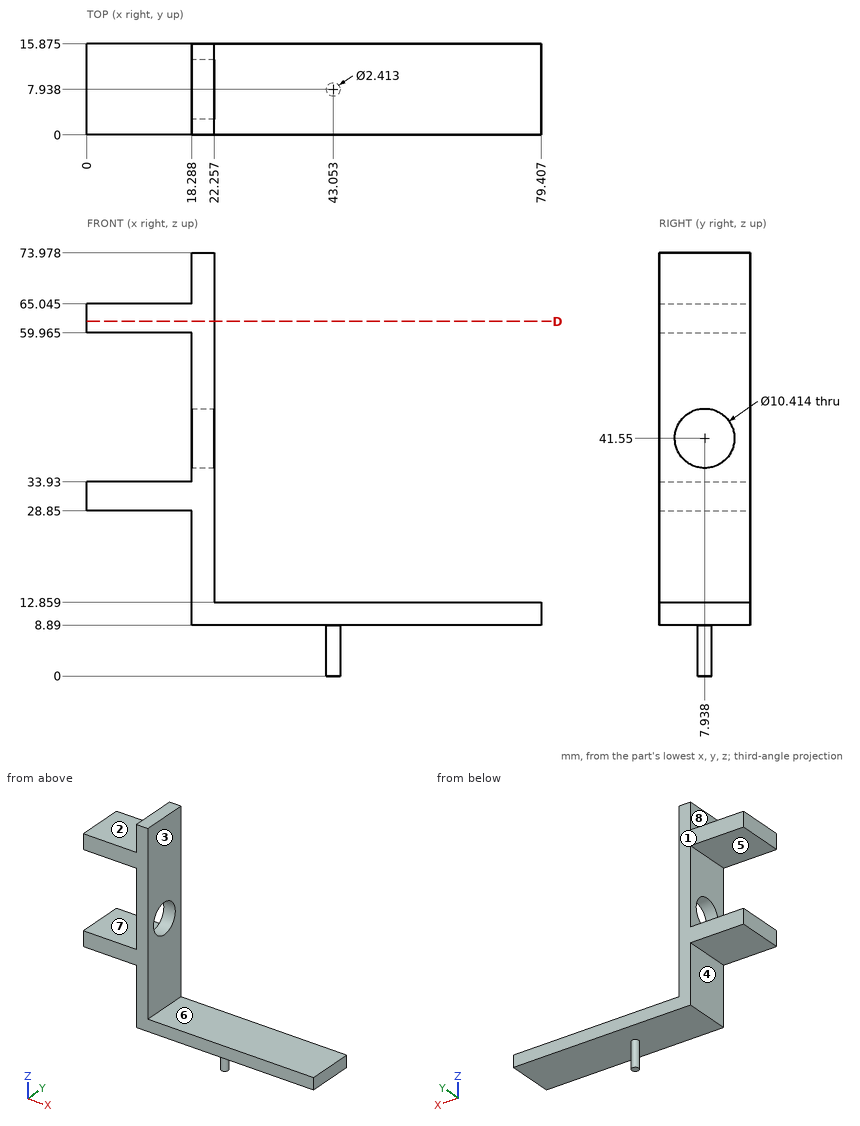
Design review of the part shown in the three views and the two pictorial views. Dimensions are in mm from the part's minimum x, y and z. A direction names the side the tool comes from. Round coordinates to 2 decimals unless told otherwise and drop trailing zeros. Loops run counter-clockwise (first coordinate to the right, second up) from the corner with the lowest first, then second, coordinate; pieces in that order, holes last. Notation, with made-up numbers: (19.5, 79) - (65.5, 79) arc R10 ccw to (65.5, 88) - close; hole circle Ø1 at (78, 11.5). An arc over 180 degrees is marked (long way). Write each question's results on one line, items separated by ' | '. Start each with the question number.
Q1. Wall thickness on line 1 along Z through (x, y) = (34.5, 7.5); line 2 along X through (y, z) = (13, 23); line 3 along Z through (x, y) = (21, 14): over which ranges is each line inside the solid? List them lowest first. Write a range as [from, to].
Q2. Insertion check: P1, Ø8, axis at y = 10, z = 47.5, coming from the -X side; P2, Ø1.5, axis at x = 31, y = 12.5, coming from the -Z side; P3, Ø2, axis at x = 56, y = 4, coming from the +Z side. Each pin has a flat end and moves straight along its axis. Give the tip position at first contact, or say it passes through.
Q3. Take a section at D-D on z = 62. Give the boundary of the cut face in (x, y) (1 decimal), plus the area to 3 significant figures.
Q4. Tool access review of the marked faces 1, 2, 3, 4 and 5: name each direction out of +Z, -Z, +X, -X, +Y, -Y from which nothing blocks a thin tool from reaching the whole face with its end or side.
Q5. Draft analysis for pull direction Z (two halves, no side actions). For the marked faces 6, 7 and 8, state which applies: pulls with the +Z half, pulls with the -Z half, needs draft (parallel to the pull), parting line crosses it, or undercut.
Data:
1) line 1: z = [8.89, 12.86] | line 2: x = [18.29, 22.26] | line 3: z = [8.89, 73.98]
2) P1: stops at x = 18.29 | P2: stops at z = 8.89 | P3: stops at z = 12.86
3) outline: (0, 0) - (22.3, 0) - (22.3, 15.9) - (0, 15.9) - close | area: 353 mm²
4) face 1: +Z, -Z, +X, -X, +Y | face 2: +Z, -X, +Y, -Y | face 3: +Z, +X, +Y, -Y | face 4: -Z, -X, +Y, -Y | face 5: -X, +Y, -Y
5) face 6: pulls with the +Z half | face 7: undercut | face 8: needs draft
